Model file for the job. Use its own axes, mm. Coordinates: 2 decimals unless noted, no trailing zeros. Order: outer loops, then holes, each group sorted by start corner. A loop starts at its lowest first (then second) coordinate and runs counter-clockwise, first axis right, second up.
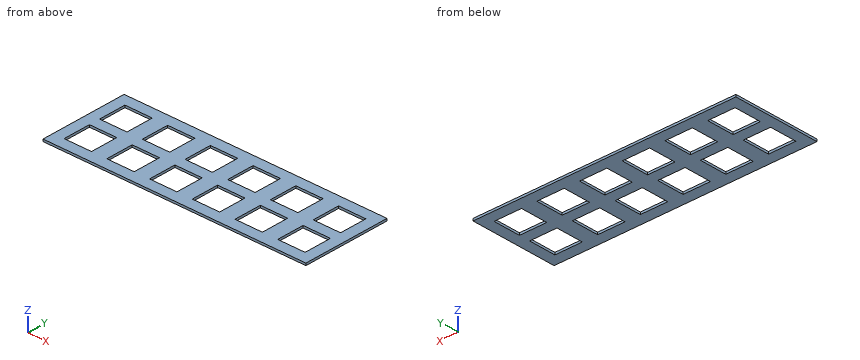
from build123d import *

# Parameters (mm, degrees)
F0_W     = 120
F0_H     = 40
F0_W_2   = 12.5
F0_H_2   = 12.5
F1_DEPTH = 1


with BuildPart() as f1:
    # F0 (on Top) → F1 (new body)
    with BuildSketch(Plane.XY):
        Rectangle(F0_W, F0_H)
        with Locations((-48.75, -8.75)):
            Rectangle(F0_W_2, F0_H_2, mode=Mode.SUBTRACT)
        with Locations((-29.25, -8.75)):
            Rectangle(F0_W_2, F0_H_2, mode=Mode.SUBTRACT)
        with Locations((-9.75, -8.75)):
            Rectangle(F0_W_2, F0_H_2, mode=Mode.SUBTRACT)
        with Locations((9.75, -8.75)):
            Rectangle(F0_W_2, F0_H_2, mode=Mode.SUBTRACT)
        with Locations((29.25, -8.75)):
            Rectangle(F0_W_2, F0_H_2, mode=Mode.SUBTRACT)
        with Locations((48.75, -8.75)):
            Rectangle(F0_W_2, F0_H_2, mode=Mode.SUBTRACT)
        with Locations((-48.75, 8.75)):
            Rectangle(F0_W_2, F0_H_2, mode=Mode.SUBTRACT)
        with Locations((-29.25, 8.75)):
            Rectangle(F0_W_2, F0_H_2, mode=Mode.SUBTRACT)
        with Locations((-9.75, 8.75)):
            Rectangle(F0_W_2, F0_H_2, mode=Mode.SUBTRACT)
        with Locations((9.75, 8.75)):
            Rectangle(F0_W_2, F0_H_2, mode=Mode.SUBTRACT)
        with Locations((29.25, 8.75)):
            Rectangle(F0_W_2, F0_H_2, mode=Mode.SUBTRACT)
        with Locations((48.75, 8.75)):
            Rectangle(F0_W_2, F0_H_2, mode=Mode.SUBTRACT)
    extrude(amount=F1_DEPTH)


solid = f1.part
Q1. Cut at A-A, the plane x = 45. List the corners of the cut face in (y, z).
Established:
outline: (-20, 0) - (-15, 0) - (-15, 1) - (-20, 1) - close; (-2.5, 0) - (2.5, 0) - (2.5, 1) - (-2.5, 1) - close; (15, 0) - (20, 0) - (20, 1) - (15, 1) - close
Q2. Probe line 1 (Y direction, x = 50, z = 0.85). List the from-to ranges inside material, lowest first.
Established:
line 1: y = -20 to -15, -2.5 to 2.5, 15 to 20
Q3. Cut at B-B, the plane y = -6.5. List the corners of the cut face in (x, z), plus the area to 3 significant figures.
Established:
outline: (-60, 0) - (-55, 0) - (-55, 1) - (-60, 1) - close; (-42.5, 0) - (-35.5, 0) - (-35.5, 1) - (-42.5, 1) - close; (-23, 0) - (-16, 0) - (-16, 1) - (-23, 1) - close; (-3.5, 0) - (3.5, 0) - (3.5, 1) - (-3.5, 1) - close; (16, 0) - (23, 0) - (23, 1) - (16, 1) - close; (35.5, 0) - (42.5, 0) - (42.5, 1) - (35.5, 1) - close; (55, 0) - (60, 0) - (60, 1) - (55, 1) - close
area: 45.0 mm2
Q4. Cut at C-C, the plane z = 0.8. Count the separate pieces of the cut face and the enclosed holes in it, plus the area to 4 significant figures.
Established:
separate pieces: 1
enclosed holes: 12
area: 2,925 mm2
